Autodesk Inventor part; units mm, degrees
ref_plane "YZ Plane" through (0, 0, 0) normal (1, 0, 0) x (0, 1, 0)
ref_plane "XZ Plane" through (0, 0, 0) normal (0, 1, 0) x (-1, 0, 0)
ref_plane "XY Plane" through (0, 0, 0) normal (0, 0, 1) x (1, 0, 0)
sketch "Sketch1" plane through (0, 0, 0) normal (0, 1, 0) x (-1, 0, 0)
  circle A0 centre (0, 0) radius 1.5
  dimension "d0" = 3
extrude "Extrusion1" add sketch "Sketch1" along normal blind 25
sketch "Sketch2" plane through (0, 25, 0) normal (0, 1, 0) x (1, 0, 0)
  circle A0 centre (0, 0) radius 1.5
extrude "Extrusion2" add sketch "Sketch2" along normal blind 2
sketch "Sketch3" plane through (0, 27, 0) normal (0, 1, 0) x (1, 0, 0)
  circle A0 centre (0, 0) radius 1.5
extrude "Extrusion3" cut sketch "Sketch3" against normal blind 1
sketch "Sketch4" plane through (0, 0, 0) normal (0, -1, 0) x (1, 0, 0)
  circle A0 centre (0, 0) radius 1.5
extrude "Extrusion4" cut sketch "Sketch4" against normal blind 1
sketch "Sketch5" plane through (0, 1, 0) normal (0, -1, 0) x (1, 0, 0)
  circle A0 centre (0, 0) radius 1
  circle A1 centre (0, 0) radius 1.5
  circle A2 centre (0, 0) radius 1.5
  dimension "d9" = 2
extrude "Extrusion5" cut sketch "Sketch5" against normal blind 1.5
fillet "Fillet1" radius 1 1 edges at (-1, 1, 0)
sketch "Sketch6" plane through (0, 26, 0) normal (0, 1, 0) x (1, 0, 0)
  circle A0 centre (0, 0) radius 1.5
  circle A1 centre (0, 0) radius 1
extrude "Extrusion6" cut sketch "Sketch6" against normal blind 2
fillet "Fillet2" radius 1 1 edges at (-1, 26, 0)
sketch "Sketch7" plane through (0, 24, 0) normal (0, 1, 0) x (1, 0, 0)
  circle A0 centre (0, 0) radius 1.5
  dimension "d16" = 3
extrude "Extrusion7" add sketch "Sketch7" along normal blind 0.5
sketch "Sketch8" plane through (0, 2.5, 0) normal (0, -1, 0) x (1, 0, 0)
  circle A0 centre (0, 0) radius 1.5
extrude "Extrusion8" cut sketch "Sketch8" along normal blind 5.5 and the other way blind 11
sketch "Sketch9" plane through (0, 13.5, 0) normal (0, -1, 0) x (1, 0, 0)
  circle A0 centre (0, 0) radius 1
  circle A1 centre (0, 0) radius 1.5
extrude "Extrusion9" cut sketch "Sketch9" against normal blind 4
sketch "Sketch10" plane through (0, 13.5, 0) normal (0, -1, 0) x (1, 0, 0)
  circle A0 centre (0, 0) radius 1
extrude "Extrusion10" add sketch "Sketch10" along normal blind 1
sketch "Sketch11" plane through (0, 12.5, 0) normal (0, -1, 0) x (1, 0, 0)
  circle A0 centre (0, 0) radius 1
extrude "Extrusion11" cut sketch "Sketch11" against normal blind 2
sketch "Sketch12" plane through (0, 14.5, 0) normal (0, -1, 0) x (1, 0, 0)
  circle A0 centre (0, 0) radius 1
extrude "Extrusion12" add sketch "Sketch12" along normal blind 1
properties part number "Pin2"
Input: part model. Units: mm. Frame: model coordinates. A direction names the side the tool comes from. Round coordinates to 2 decimals unless told otherwise and drop trailing zeros. Write each loop counter-clockwise with the first axis right and the second up, starting at its lowest first coordinate (ties: lowest second). Pieces come first, ordered by that corner, then holes. Notation, with made-up numbers: (12, 61.25) - (48, 61.25) arc R24 ccw to (48, 80.25) - close; hole circle Ø2 at (33.5, 36.25). An arc over 180 degrees is marked (long way). Write item = value, one per line.
(1) Contact query for a flat-ended pin moving along its axis: pin 1 Ø1 at (y, z) = (19.5, 1) entering from -X. Output: stop coordinate, or through.
Geometry check:
pin_1 = -1.41
(2) Material intervals for probe 1 along Y at (x, z) = (-0.35, 1.35); probe 2 along Y at (x, z) = (-0.35, -0.4); probe 3 along Z at (x, y) = (-1.05, 20.75), sorted ascending.
Geometry check:
probe_1 = 17.5 to 24.5
probe_2 = 13.5 to 25.85
probe_3 = -1.07 to 1.07
(3) Section query C-C on y = 16. Output: boundary loops of the cut face in (x, z).
Geometry check:
outline = circle Ø2 at (0, 0)
(4) Access query for faces 1 (the cylindrical face through (0, 16, 1)), 2 (the cylindrical face through (-0.217, 24.754, 0.976)), 3 (the flat face through (0, 13.5, 0)). Directions: +Z, -Z, +X, -X, +Y, -Y. A direction counts if a zero-diameter tool reaches every point of the face in a straight line with its end or side. Return the directions, or none.
Geometry check:
face_1 = -Y
face_2 = +Y
face_3 = +Z, -Z, +X, -X, -Y
(5) Section query A-A on z = -0.15. Output: boundary loops of the cut face in (x, y).
Geometry check:
outline = (-1.49, 17.5) - (-0.99, 17.5) - (-0.99, 13.5) - (0.99, 13.5) - (0.99, 17.5) - (1.49, 17.5) - (1.49, 24.5) - (0.99, 24.5) - (0.99, 25) arc R0.99 ccw to (-0.99, 25) - (-0.99, 24.5) - (-1.49, 24.5) - close
(6) Section query B-B on y = 20. Output: boundary loops of the cut face in (x, z).
Geometry check:
outline = circle Ø3 at (0, 0)
